```python
from build123d import *

# Parameters (mm, degrees)
BOSS_EXTRUDE1_DEPTH     = 20
CUT_EXTRUDE1_DEPTH      = 22.213203436
CUT_EXTRUDE1_DEPTH_BACK = 22.213203436
CUT_EXTRUDE2_DEPTH      = 22.213203436
SKETCH4_R               = 2.375
BOSS_EXTRUDE2_DEPTH     = 1.375
SKETCH5_R               = 2.625
CUT_EXTRUDE3_DEPTH      = 24.327156921
SKETCH6_R               = 2.625
CUT_EXTRUDE4_DEPTH      = 1.625
BOSS_EXTRUDE3_REACH     = 25.397
SKETCH7_R               = 2.375
BOSS_EXTRUDE4_START     = -3.375
SKETCH8_R               = 2.375
BOSS_EXTRUDE4_DEPTH     = 3.375
CUT_EXTRUDE5_DEPTH      = 24.327156921
CUT_EXTRUDE5_DEPTH_BACK = 24.327156921
SKETCH10_R              = 1.45
CUT_EXTRUDE6_DEPTH      = 25.566555009
CUT_EXTRUDE6_DEPTH_BACK = 25.566555009
SKETCH11_R              = 1.45


with BuildPart() as part:
    # Sketch1 → Boss-Extrude1 (new body)
    with BuildSketch(Plane(origin=(0, 0, 0), x_dir=(1, 0, 0), z_dir=(0, 1, 0))):
        Polygon((-1.666666667, -5), (1.666666667, -5), (5, -1.666666667), (5, 1.666666667), (1.666666667, 5), (-1.666666667, 5), (-5, 1.666666667), (-5, -1.666666667), align=None)
    extrude(amount=BOSS_EXTRUDE1_DEPTH)

    # Sketch2 → Cut-Extrude1 (cut, two sides: drawn at the far end of the back side and taken through both)
    with BuildSketch(Plane(origin=(0, 0, 0), x_dir=(0, 0, -1), z_dir=(1, 0, 0)).offset(-CUT_EXTRUDE1_DEPTH_BACK)):
        Polygon((0, 20), (-5, 20), (-5, 15), align=None)
        Polygon((0, 0), (-5, 0), (-5, 5), align=None)
    extrude(amount=CUT_EXTRUDE1_DEPTH + CUT_EXTRUDE1_DEPTH_BACK, mode=Mode.SUBTRACT)

    # Sketch3 → Cut-Extrude2 (cut, through all)
    with BuildSketch(Plane(origin=(0, 0, 0), x_dir=(1, 0, 0), z_dir=(0, 1, 0))):
        Polygon((0, -4.5), (-0.5, -4), (-0.5, -3.5), (0.5, -3.5), (0.5, -4), align=None)
        Polygon((0.5, 4.5), (0.5, 4), (0, 3.5), (-0.5, 4), (-0.5, 4.5), align=None)
    extrude(amount=CUT_EXTRUDE2_DEPTH, mode=Mode.SUBTRACT)

    # Sketch4 → Boss-Extrude2 (add, symmetric)
    with BuildSketch(Plane(origin=(0, 0, 0), x_dir=(0, 0, -1), z_dir=(1, 0, 0))):
        with Locations((0, 19.5)):
            Circle(SKETCH4_R)
    extrude(amount=BOSS_EXTRUDE2_DEPTH, both=True)

    # Sketch5 → Cut-Extrude3 (cut, through all)
    with BuildSketch(Plane(origin=(1.375, 0, 0), x_dir=(0, 0, -1), z_dir=(1, 0, 0))):
        with Locations((0, 19.5)):
            Circle(SKETCH5_R)
    cut_extrude3 = extrude(amount=CUT_EXTRUDE3_DEPTH, mode=Mode.SUBTRACT)

    # Mirror1: Cut-Extrude3 across plane
    add(cut_extrude3.mirror(Plane(origin=(0, 0, 0), x_dir=(0, 0, 1), z_dir=(1, 0, 0))), mode=Mode.SUBTRACT)

    # Sketch6 → Cut-Extrude4 (cut, symmetric)
    with BuildSketch(Plane(origin=(0, 0, 0), x_dir=(0, 0, -1), z_dir=(1, 0, 0))):
        with Locations((0, -0.5)):
            Circle(SKETCH6_R)
    extrude(amount=CUT_EXTRUDE4_DEPTH, both=True, mode=Mode.SUBTRACT)

    # Boss-Extrude3: up to this face of the body (flat: up to its plane)
    boss_extrude3_end = Plane(part.part.faces().sort_by_distance((-5, 8.732537251, -0.027810101))[0])
    # Sketch7 → Boss-Extrude3 (add, up to the picked face)
    with BuildSketch(Plane(origin=(-1.625, 0, 0), x_dir=(0, 0, -1), z_dir=(1, 0, 0)), mode=Mode.PRIVATE) as boss_extrude3_sk1:
        with Locations((0, -0.5)):
            Circle(SKETCH7_R)
    boss_extrude3_tool1 = split(extrude(boss_extrude3_sk1.sketch, amount=-BOSS_EXTRUDE3_REACH, mode=Mode.PRIVATE), bisect_by=boss_extrude3_end, keep=Keep.BOTH, mode=Mode.PRIVATE)
    add(boss_extrude3_tool1.solids().sort_by(Axis((-1.625, -0.5, 0), (-1, 0, 0)))[0])

    # Sketch8 → Boss-Extrude4 (add)
    with BuildSketch(Plane.ZY.offset(-1.625).offset(BOSS_EXTRUDE4_START)):
        with Locations((0, -0.5)):
            Circle(SKETCH8_R)
    extrude(amount=BOSS_EXTRUDE4_DEPTH)

    # Sketch10 → Cut-Extrude5 (cut, two sides: drawn at the far end of the back side and taken through both)
    with BuildSketch(Plane(origin=(1.375, 0, 0), x_dir=(0, 0, -1), z_dir=(1, 0, 0)).offset(-CUT_EXTRUDE5_DEPTH_BACK)):
        with Locations((0, 19.5)):
            Circle(SKETCH10_R)
    extrude(amount=CUT_EXTRUDE5_DEPTH + CUT_EXTRUDE5_DEPTH_BACK, mode=Mode.SUBTRACT)

    # Sketch11 → Cut-Extrude6 (cut, two sides: drawn at the far end of the back side and taken through both)
    with BuildSketch(Plane(origin=(5, 0, 0), x_dir=(0, 0, -1), z_dir=(1, 0, 0)).offset(-CUT_EXTRUDE6_DEPTH_BACK)):
        with Locations((0, -0.5)):
            Circle(SKETCH11_R)
    extrude(amount=CUT_EXTRUDE6_DEPTH + CUT_EXTRUDE6_DEPTH_BACK, mode=Mode.SUBTRACT)


solid = part.part
```
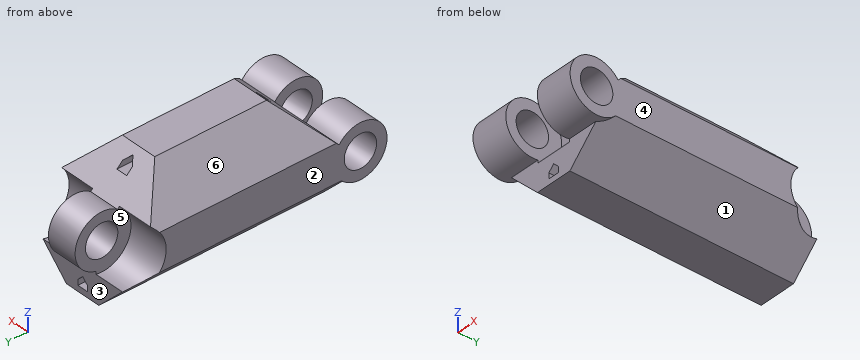
Design review of the part built by this model. Coordinates are the model's own, in mm. Face numbers are marked on the shaded views. A direction names the side the tool comes from. Round coordinates to 2 decimals unless told otherwise and drop trailing zeros. Write each loop counter-clockwise with the first axis right and the second up, starting at its lowest first coordinate (ties: lowest second). Pieces come first, ordered by that corner, then holes. Notation, with made-up numbers: (7, 0) -> (24, 0) arc R31 ccw to (24, 38) -> close; hole circle Ø3 at (21.25, -2). An arc over 180 degrees is marked (long way). Answer in a Markdown table with one row per item.
Q1. Take a section at B-B, the plane y = 10. State the section outline as (x, z) points, then the cut area to 3 significant figures.
The answers:
| item | result |
|---|---|
| outline | (-5, -1.67) -> (-1.67, -5) -> (1.67, -5) -> (5, -1.67) -> (5, 1.67) -> (1.67, 5) -> (-1.67, 5) -> (-5, 1.67) -> close; hole (-0.5, -4.5) -> (0.5, -4.5) -> (0.5, -4) -> (0, -3.5) -> (-0.5, -4) -> close; hole (-0.5, 3.5) -> (0.5, 3.5) -> (0.5, 4) -> (0, 4.5) -> (-0.5, 4) -> close |
| area | 76.3 mm² |
Q2. For the marked faces 1, 2 and 3, list the 3-axis set-ups (+Z, -Z, +X, -X, +Y, -Y) from which the entire face can be reached by the end or side of a thin tool; tool diameter is ignored.
The answers:
| item | result |
|---|---|
| face 1 | -Z, +X, +Y |
| face 2 | +Z, -Z, -X, +Y, -Y |
| face 3 | -Z, +X, -X, +Y |
Q3. Draft analysis for pull direction Z (two halves, no side actions). For the marked faces 4, 5 and 6, state which applies: +Z half, -Z half, draft (parallel to the pull), parting line (faces both ways), or undercut.
The answers:
| item | result |
|---|---|
| face 4 | draft |
| face 5 | undercut |
| face 6 | +Z half |
Q4. Take a section at A-A, the plane z = 0. State the section outline as (x, y) points (3 decimals), then the cut area to 3 significant figures.
The answers:
| item | result |
|---|---|
| outline | (-5, -2.875) -> (-1.625, -2.875) -> (-1.625, -1.95) -> (-5, -1.95) -> close; (-5, 0.95) -> (-1.625, 0.95) -> (-1.625, 2.125) -> (1.625, 2.125) -> (1.625, 0.95) -> (5, 0.95) -> (5, 16.875) -> (1.375, 16.875) -> (1.375, 18.05) -> (-1.375, 18.05) -> (-1.375, 16.875) -> (-5, 16.875) -> close; (-1.375, 20.95) -> (1.375, 20.95) -> (1.375, 21.875) -> (-1.375, 21.875) -> close; (1.625, -2.875) -> (5, -2.875) -> (5, -1.95) -> (1.625, -1.95) -> close |
| area | 167 mm² |
Q5. Take a section at D-D, the plane x = -2.75. State the section outline as (y, z) points (3 decimals), then the cut area to 3 significant figures.
The answers:
| item | result |
|---|---|
| outline | (0, -3.917) -> (20, -3.917) -> (20, -2.577) arc R2.625 cw to (17.911, 2.089) -> (16.083, 3.917) -> (3.917, 3.917) -> (1.411, 1.411) arc R2.375 ccw (long way) to (0, -2.322) -> close; hole circle Ø2.9 at (-0.5, 0) |
| area | 137 mm² |
Q6. To check wall thickness, follow L1, parallel to Z at x = -3.25, y = -0.5 (3 decimals); L2, parallel to Y at x = -0.2, z = 0 (3 decimals); L3, parallel to Y at x = 4.05, z = 0 (3 decimals). State the ranges of each line that lie inside material, in increasing order. Write a range as [from, to].
The answers:
| item | result |
|---|---|
| L1 | [-2.375, -1.45], [1.45, 2.375] |
| L2 | [2.125, 18.05], [20.95, 21.875] |
| L3 | [-2.875, -1.95], [0.95, 16.875] |
Q7. Take a section at C-C, the plane y = -0.5. State the section outline as (x, z) points (3 decimals), then the cut area to 3 significant figures.
The answers:
| item | result |
|---|---|
| outline | (-5, -2.375) -> (-1.625, -2.375) -> (-1.625, -1.45) -> (-5, -1.45) -> close; (-5, 1.45) -> (-1.625, 1.45) -> (-1.625, 2.375) -> (-5, 2.375) -> close; (1.625, -2.375) -> (5, -2.375) -> (5, -1.45) -> (1.625, -1.45) -> close; (1.625, 1.45) -> (5, 1.45) -> (5, 2.375) -> (1.625, 2.375) -> close |
| area | 12.5 mm² |
Q8. Clearance check with flat-ended pins moving along their axes: pin 1 Ø5 at (x, y) = (1.5, 2) entering from +Z; pin 2 Ø0.6 at (y, z) = (12, 3.5) entering from +X; pin 3 Ø0.8 at (x, z) = (-1.5, -3) entering from +Y; pin 4 Ø2.5 at (y, z) = (-0.5, 0) entering from -X. State where each tip first meets the part, or that it passes through.
The answers:
| item | result |
|---|---|
| pin 1 | z = 4.5 |
| pin 2 | x = 3.47 |
| pin 3 | y = 20 |
| pin 4 | through |
